```python
from build123d import *

# Parameters (mm, degrees)
F3_R = 5


with BuildPart() as f1:
    # F0 (on Front) → F1 (revolve)
    with BuildSketch(Plane.XZ):
        Polygon((0, 13.1249994196), (0, 0), (125.5859370285, 0), (125.5859370285, 17.5), (85.5859370285, 17.5), (85.5859370285, 30), (70.546875798, 30), (41.5774360299, 13.1249994196), (31.0279354453, 13.1249994196), (31.0279354453, 43.1288294494), (25.7531870157, 43.1288294494), (25.7531870157, 13.1249994196), (20.168159157, 13.1249994196), (20.168159157, 32.8896120191), (15.2036882937, 32.8896120191), (15.2036882937, 13.1249994196), (9.6186613664, 13.1249994196), (9.6186613664, 22.3401114345), (5.5850301869, 22.3401114345), (5.5850301869, 13.1249994196), align=None)
    revolve(axis=Axis((62.7929685142, 0, 0), (-1, 0, 0)))

    # F2: F1 across face


with BuildPart() as f1_1:
    add(f1.part)
    add(f1.part.mirror(Plane(origin=(0, 0, 0), x_dir=(0, -1, 0), z_dir=(-1, 0, 0))))

    # F3
    f3_edges = [f1_1.edges().sort_by_distance(p)[0] for p in [
        (-85.585937, 0, -30),
        (85.585937, 0, -30),
        (125.585937, 0, -17.5),
        (-125.585937, 0, -17.5),
    ]]
    fillet(f3_edges, radius=F3_R)


solid = f1_1.part
```
The model under review builds one solid part; all positions refer to its coordinate system, in mm. A direction names the side the tool comes from. Round coordinates to 2 decimals unless told otherwise and drop trailing zeros. Write each loop counter-clockwise with the first axis right and the second up, starting at its lowest first coordinate (ties: lowest second). Pieces come first, ordered by that corner, then holes. Notation, with made-up numbers: M -31,16 L -13,16 A18 cw -13,23 Z; hole C 51,21 d2. An arc over 180 degrees is marked long. Use CSV: the item, a comma, the result in double quotes. Start each with the question number.
(1) We need section B-B, the plane x = 56.5. State the section outline as (y, z) points.
(2) For line 1 along X through (y, z) = (27, -24); line 2 along X through (y, z) = (-12, 28.5); line 3 along X through (y, z) = (25, 4.5), list the stretches that pass through material, from the lowest coordinate up.
(3) We need section A-A, the plane x = 93. State the section outline as (y, z) points.
(4) Tool access review of faces 5 (the face through (46.2, -15.44, -3.43)), 6 (the face through (-85.586, -5, 17)): name each direction out of +Z, -Z, +X, -X, +Y, -Y from which nothing blocks a thin tool from reaching the whole face with its end or side.
(5) Clearance check with flat-ended pins moving along their axes: P1, Ø5, axis at x = 16, z = 32, coming from the +Y side; P2, Ø8, axis at x = 73.5, z = 30.5, coming from the -Y side; P3, Ø3, axis at x = 60, z = 20.5, coming from the +Y side. State where each tip first meets the part, or that it passes through.
(6) The part is to be moulded in two halves that separate along X. For faces 1 (the face through (125.586, 0, 0)), 2 (the face through (25.753, -9, -10)), 3 (the face through (-125.586, 0, 0)), 4 (the face through (28.354, 36.366, 23.186)), say which applies: +X half, -X half, draft (parallel to the pull), parting line (faces both ways), or undercut.
Findings:
1,outline,"C 0,0 d43.64"
2,line 1,"-31.03 to -25.75, 25.75 to 31.03"
2,line 2,"-31.03 to -25.75, -20.17 to -15.2, 15.2 to 20.17, 25.75 to 31.03"
2,line 3,"-85.57 to -62.65, -31.03 to -25.75, -20.17 to -15.2, 15.2 to 20.17, 25.75 to 31.03, 62.65 to 85.57"
3,outline,"C 0,0 d35"
4,face 5,"none"
4,face 6,"-X"
5,P1,"y = 14.54"
5,P2,"y = -14.06"
5,P3,"y = 14.9"
6,face 1,"+X half"
6,face 2,"undercut"
6,face 3,"-X half"
6,face 4,"draft"
